```python
from build123d import *

# Parameters (mm, degrees)
BOSS_EXTRUDE1_OUTLINE_R = 9
BOSS_EXTRUDE1_DEPTH     = 1.5
SKETCH2_R               = 6.1121977
BOSS_EXTRUDE2_DEPTH     = 5.5
SKETCH3_R               = 2.5
CUT_EXTRUDE1_DEPTH      = 19.920887928
SKETCH4_R               = 5.6
SKETCH4_R_2             = 5.5
SKETCH4_R_3             = 4.5
SKETCH4_R_4             = 3.5
CUT_EXTRUDE2_DEPTH      = 0.5


# Read off the part's stored shape, not the designer's step: Boss-Extrude1
with BuildPart() as part:
    # Boss-Extrude1 outline → Boss-Extrude1 (new body)
    with BuildSketch(Plane(origin=(0, 0, 0), x_dir=(1, 0, 0), z_dir=(0, 1, 0))):
        Circle(BOSS_EXTRUDE1_OUTLINE_R)
    boss_extrude1 = extrude(amount=BOSS_EXTRUDE1_DEPTH)

    # Sketch2 → Boss-Extrude2 (add)
    with BuildSketch(Plane(origin=(0, 1.5, 0), x_dir=(1, 0, 0), z_dir=(0, 1, 0))):
        with Locations(Location((0, 0, 0), (0, 0, 270))):
            Circle(SKETCH2_R)
    boss_extrude2 = extrude(amount=BOSS_EXTRUDE2_DEPTH)

    # Mirror1: Boss-Extrude2 across plane
    add(boss_extrude2.mirror(Plane.ZX.offset(7)))

    # Mirror2: Boss-Extrude1 across plane
    add(boss_extrude1.mirror(Plane.ZX.offset(7)))

    # Sketch3 → Cut-Extrude1 (cut, through all)
    with BuildSketch(Plane(origin=(0, 14, 0), x_dir=(1, 0, 0), z_dir=(0, 1, 0))):
        with Locations(Location((0, 0, 0), (0, 0, 270))):
            Circle(SKETCH3_R)
    extrude(amount=-CUT_EXTRUDE1_DEPTH, mode=Mode.SUBTRACT)

    # Sketch4 → Cut-Extrude2 (cut)
    # profile 1 of 2: a face of its own
    with BuildSketch(Plane(origin=(0, 14, 0), x_dir=(1, 0, 0), z_dir=(0, 1, 0))):
        with Locations(Location((0, 0, 0), (0, 0, 270))):
            Circle(SKETCH4_R)
        with Locations(Location((0, 0, 0), (0, 0, 270))):
            Circle(SKETCH4_R_2, mode=Mode.SUBTRACT)
    # profile 2 of 2: a face of its own
    with BuildSketch(Plane(origin=(0, 14, 0), x_dir=(1, 0, 0), z_dir=(0, 1, 0))):
        with Locations(Location((0, 0, 0), (0, 0, 270))):
            Circle(SKETCH4_R_3)
        with Locations(Location((0, 0, 0), (0, 0, 270))):
            Circle(SKETCH4_R_4, mode=Mode.SUBTRACT)
    cut_extrude2 = extrude(amount=-CUT_EXTRUDE2_DEPTH, mode=Mode.SUBTRACT)

    # Mirror3: Cut-Extrude2 across plane
    add(cut_extrude2.mirror(Plane.ZX.offset(7)), mode=Mode.SUBTRACT)


solid = part.part
```
Here's how the part is built. I have some questions about the finished solid (model axes, mm). A direction names the side the tool comes from. Coordinates: 2 decimals unless noted, no trailing zeros. Order: outer loops, then holes, each group sorted by start corner. A loop starts at its lowest first (then second) coordinate and runs counter-clockwise, first axis right, second up. Notation, with made-up numbers: (-36.5, 28) -> (-31.5, 28) arc R18 cw to (-31.5, 56) -> close; hole circle Ø7 at (32, 58.25). An arc over 180 degrees is marked (long way). Return JSON: item names as keys, results as strings.
1) Thinking about a two-plate mould opening in Z: for faces 1 (the cylindrical face through (-1.172, 0.74, -8.923)), 2 (the cylindrical face through (1.352, 13.754, 4.292)), 3 (the flat face through (-5, 14, 0)), 4 (the cylindrical face through (-2.44, 7.1, -0.54)), which applies, +Z half, -Z half, draft (parallel to the pull), parting line (faces both ways), or undercut?
Conclusion:
{"face 1": "parting line", "face 2": "undercut", "face 3": "draft", "face 4": "undercut"}
2) If we section it at B-B on y = 13.25: List the corners of the cut face in (x, z) for me, plus the area to 3 significant figures.
Conclusion:
{"outline": "circle Ø18 at (0, 0); hole circle Ø5 at (0, 0)", "area": "235 mm²"}
3) If we section it at D-D on y = 10.5: List the corners of the cut face in (x, z) for me.
Conclusion:
{"outline": "circle Ø12.22 at (0, 0); hole circle Ø5 at (0, 0)"}
4) If we section it at C-C on z = 7.25: List the corners of the cut face in (x, y) for me, plus the area to 3 significant figures.
Conclusion:
{"outline": "(-5.33, 0) -> (5.33, 0) -> (5.33, 1.5) -> (-5.33, 1.5) -> close; (-5.33, 12.5) -> (5.33, 12.5) -> (5.33, 14) -> (-5.33, 14) -> close", "area": "32.0 mm²"}
5) If I drill on probe 1 along Y at (x, z) = (6.5, 5.5); probe 2 along X at (y, z) = (7.5, 0); probe 3 along Y at (x, z) = (4, 2), over which ranges is the centre line in solid material (lowest first)?
Conclusion:
{"probe 1": "y = 0 to 1.5, 12.5 to 14", "probe 2": "x = -6.11 to -2.5, 2.5 to 6.11", "probe 3": "y = 0.5 to 13.5"}
6) On a 3-axis mill with a long thin cutter (end or side, diameter ignored), from which of +Z, -Z, +X, -X, +Y, -Y can I reach the whole of each face in a straight line? I mean faces 5 (the cylindrical face through (-3.417, 13.754, -0.759)), 6 (the cylindrical face through (1.352, 0.246, 4.292)), 7 (the flat face through (2, 1.5, 6)), 8 (the cylindrical face through (-1.172, 13.26, -8.923)), 9 (the flat face through (-5, 0, 0)). Say none if no direction works.
Conclusion:
{"face 5": "+Y", "face 6": "-Y", "face 7": "none", "face 8": "+Y, -Y", "face 9": "+Z, -Z, +X, -X, -Y"}
7) If we section it at A-A on x = 7.75: List the corners of the cut face in (y, z) for me.
Conclusion:
{"outline": "(0, -4.58) -> (1.5, -4.58) -> (1.5, 4.58) -> (0, 4.58) -> close; (12.5, -4.58) -> (14, -4.58) -> (14, 4.58) -> (12.5, 4.58) -> close"}
8) I'm going to push flat-ended pins straight in: P1, Ø6, axis at x = -4.5, y = 2, coming from the +Z side; P2, Ø9, axis at x = 0, z = 0, coming from the -Y side; P3, Ø6, axis at x = 6, y = 7.5, coming from the +Z side; P4, Ø3, axis at y = 6, z = -3.5, coming from the +X side. Where does each tip first touch, or does it pass through?
Conclusion:
{"P1": "stops at z = 8.87", "P2": "stops at y = 0", "P3": "stops at z = 5.33", "P4": "stops at x = 5.78"}
